from build123d import *

# Parameters (mm, degrees)
F0_R     = 2.157429
F0_R_2   = 5.60947
F1_DEPTH = 3.175
F2_DEPTH = 0.004921
F3_DEPTH = 3.175


with BuildPart() as f1:
    # F0 (on Front) → F1 (new body)
    with BuildSketch(Plane.XZ):
        with BuildLine():
            Line((19.481216, 38.301506), (-40.142396, 38.301506))
            ThreePointArc((-40.142396, 38.301506), (-44.686392, 36.387111), (-46.490546, 31.798229))
            Line((-46.490546, 31.798229), (-44.625234, 18.579618))
            ThreePointArc((-44.625234, 18.579618), (-43.776004, 17.017098), (-42.110151, 16.394528))
            Line((-42.110151, 16.394528), (21.620648, 16.394528))
            ThreePointArc((21.620648, 16.394528), (23.297675, 17.026865), (24.139706, 18.609033))
            Line((24.139706, 18.609033), (25.823629, 31.641185))
            ThreePointArc((25.823629, 31.641185), (24.07975, 36.330545), (19.481216, 38.301506))
        make_face()
        with Locations((-36.75957, 20.633117)):
            Circle(F0_R, mode=Mode.SUBTRACT)
        with Locations((17.996946, 20.940602)):
            Circle(F0_R, mode=Mode.SUBTRACT)
        with Locations((-38.274463, 31.951506)):
            Circle(F0_R_2, mode=Mode.SUBTRACT)
        with BuildLine():
            Line((-29.799683, 20.633117), (-29.799683, 34.853889))
            ThreePointArc((-29.799683, 34.853889), (-27.878732, 36.660702), (-26.0331, 34.777018))
            Line((-26.0331, 34.777018), (-26.0331, 20.556246))
            ThreePointArc((-26.0331, 20.556246), (-27.954051, 18.749433), (-29.799683, 20.633117))
        make_face(mode=Mode.SUBTRACT)
        with BuildLine():
            Line((-24.176236, 20.709988), (-24.176236, 34.93076))
            ThreePointArc((-24.176236, 34.93076), (-22.255285, 36.737572), (-20.409653, 34.853889))
            Line((-20.409653, 34.853889), (-20.409653, 20.633116))
            ThreePointArc((-20.409653, 20.633116), (-22.330604, 18.826304), (-24.176236, 20.709988))
        make_face(mode=Mode.SUBTRACT)
        with BuildLine():
            Line((-18.419787, 20.786859), (-18.419787, 35.007631))
            ThreePointArc((-18.419787, 35.007631), (-16.498836, 36.814444), (-14.653204, 34.93076))
            Line((-14.653204, 34.93076), (-14.653204, 20.709988))
            ThreePointArc((-14.653204, 20.709988), (-16.574155, 18.903175), (-18.419787, 20.786859))
        make_face(mode=Mode.SUBTRACT)
        with BuildLine():
            Line((-12.493486, 20.86373), (-12.493486, 35.084503))
            ThreePointArc((-12.493486, 35.084503), (-10.572535, 36.891315), (-8.726902, 35.007631))
            Line((-8.726902, 35.007631), (-8.726902, 20.786859))
            ThreePointArc((-8.726902, 20.786859), (-10.647853, 18.980047), (-12.493486, 20.86373))
        make_face(mode=Mode.SUBTRACT)
        with BuildLine():
            Line((-6.886294, 20.940602), (-6.886294, 35.161374))
            ThreePointArc((-6.886294, 35.161374), (-4.965343, 36.968187), (-3.11971, 35.084503))
            Line((-3.11971, 35.084503), (-3.11971, 20.86373))
            ThreePointArc((-3.11971, 20.86373), (-5.040661, 19.056918), (-6.886294, 20.940602))
        make_face(mode=Mode.SUBTRACT)
        with BuildLine():
            Line((-1.18931, 21.017473), (-1.18931, 35.238246))
            ThreePointArc((-1.18931, 35.238246), (0.73164, 37.045058), (2.577273, 35.161374))
            Line((2.577273, 35.161374), (2.577273, 20.940602))
            ThreePointArc((2.577273, 20.940602), (0.656322, 19.133789), (-1.18931, 21.017473))
        make_face(mode=Mode.SUBTRACT)
        with BuildLine():
            Line((4.431474, 21.017473), (4.431474, 35.238246))
            ThreePointArc((4.431474, 35.238246), (6.352424, 37.045058), (8.198057, 35.161374))
            Line((8.198057, 35.161374), (8.198057, 20.940602))
            ThreePointArc((8.198057, 20.940602), (6.277106, 19.133789), (4.431474, 21.017473))
        make_face(mode=Mode.SUBTRACT)
        with Locations((17.949626, 31.951506)):
            Circle(F0_R_2, mode=Mode.SUBTRACT)
    extrude(amount=F1_DEPTH)

    # F0 (on Front) → F2 (join)
    with BuildSketch(Plane.XZ):
        with BuildLine():
            Line((19.481216, 38.301506), (-40.142396, 38.301506))
            ThreePointArc((-40.142396, 38.301506), (-44.686392, 36.387111), (-46.490546, 31.798229))
            Line((-46.490546, 31.798229), (-44.625234, 18.579618))
            ThreePointArc((-44.625234, 18.579618), (-43.776004, 17.017098), (-42.110151, 16.394528))
            Line((-42.110151, 16.394528), (21.620648, 16.394528))
            ThreePointArc((21.620648, 16.394528), (23.297675, 17.026865), (24.139706, 18.609033))
            Line((24.139706, 18.609033), (25.823629, 31.641185))
            ThreePointArc((25.823629, 31.641185), (24.07975, 36.330545), (19.481216, 38.301506))
        make_face()
        with Locations((-36.75957, 20.633117)):
            Circle(F0_R, mode=Mode.SUBTRACT)
        with Locations((17.996946, 20.940602)):
            Circle(F0_R, mode=Mode.SUBTRACT)
        with Locations((-38.274463, 31.951506)):
            Circle(F0_R_2, mode=Mode.SUBTRACT)
        with BuildLine():
            Line((-29.799683, 20.633117), (-29.799683, 34.853889))
            ThreePointArc((-29.799683, 34.853889), (-27.878732, 36.660702), (-26.0331, 34.777018))
            Line((-26.0331, 34.777018), (-26.0331, 20.556246))
            ThreePointArc((-26.0331, 20.556246), (-27.954051, 18.749433), (-29.799683, 20.633117))
        make_face(mode=Mode.SUBTRACT)
        with BuildLine():
            Line((-24.176236, 20.709988), (-24.176236, 34.93076))
            ThreePointArc((-24.176236, 34.93076), (-22.255285, 36.737572), (-20.409653, 34.853889))
            Line((-20.409653, 34.853889), (-20.409653, 20.633116))
            ThreePointArc((-20.409653, 20.633116), (-22.330604, 18.826304), (-24.176236, 20.709988))
        make_face(mode=Mode.SUBTRACT)
        with BuildLine():
            Line((-18.419787, 20.786859), (-18.419787, 35.007631))
            ThreePointArc((-18.419787, 35.007631), (-16.498836, 36.814444), (-14.653204, 34.93076))
            Line((-14.653204, 34.93076), (-14.653204, 20.709988))
            ThreePointArc((-14.653204, 20.709988), (-16.574155, 18.903175), (-18.419787, 20.786859))
        make_face(mode=Mode.SUBTRACT)
        with BuildLine():
            Line((-12.493486, 20.86373), (-12.493486, 35.084503))
            ThreePointArc((-12.493486, 35.084503), (-10.572535, 36.891315), (-8.726902, 35.007631))
            Line((-8.726902, 35.007631), (-8.726902, 20.786859))
            ThreePointArc((-8.726902, 20.786859), (-10.647853, 18.980047), (-12.493486, 20.86373))
        make_face(mode=Mode.SUBTRACT)
        with BuildLine():
            Line((-6.886294, 20.940602), (-6.886294, 35.161374))
            ThreePointArc((-6.886294, 35.161374), (-4.965343, 36.968187), (-3.11971, 35.084503))
            Line((-3.11971, 35.084503), (-3.11971, 20.86373))
            ThreePointArc((-3.11971, 20.86373), (-5.040661, 19.056918), (-6.886294, 20.940602))
        make_face(mode=Mode.SUBTRACT)
        with BuildLine():
            Line((-1.18931, 21.017473), (-1.18931, 35.238246))
            ThreePointArc((-1.18931, 35.238246), (0.73164, 37.045058), (2.577273, 35.161374))
            Line((2.577273, 35.161374), (2.577273, 20.940602))
            ThreePointArc((2.577273, 20.940602), (0.656322, 19.133789), (-1.18931, 21.017473))
        make_face(mode=Mode.SUBTRACT)
        with BuildLine():
            Line((4.431474, 21.017473), (4.431474, 35.238246))
            ThreePointArc((4.431474, 35.238246), (6.352424, 37.045058), (8.198057, 35.161374))
            Line((8.198057, 35.161374), (8.198057, 20.940602))
            ThreePointArc((8.198057, 20.940602), (6.277106, 19.133789), (4.431474, 21.017473))
        make_face(mode=Mode.SUBTRACT)
        with Locations((17.949626, 31.951506)):
            Circle(F0_R_2, mode=Mode.SUBTRACT)
    extrude(amount=F2_DEPTH)

    # F0 (on Front) → F3 (join)
    with BuildSketch(Plane.XZ):
        with BuildLine():
            Line((19.481216, 38.301506), (-40.142396, 38.301506))
            ThreePointArc((-40.142396, 38.301506), (-44.686392, 36.387111), (-46.490546, 31.798229))
            Line((-46.490546, 31.798229), (-44.625234, 18.579618))
            ThreePointArc((-44.625234, 18.579618), (-43.776004, 17.017098), (-42.110151, 16.394528))
            Line((-42.110151, 16.394528), (21.620648, 16.394528))
            ThreePointArc((21.620648, 16.394528), (23.297675, 17.026865), (24.139706, 18.609033))
            Line((24.139706, 18.609033), (25.823629, 31.641185))
            ThreePointArc((25.823629, 31.641185), (24.07975, 36.330545), (19.481216, 38.301506))
        make_face()
        with Locations((-36.75957, 20.633117)):
            Circle(F0_R, mode=Mode.SUBTRACT)
        with Locations((17.996946, 20.940602)):
            Circle(F0_R, mode=Mode.SUBTRACT)
        with Locations((-38.274463, 31.951506)):
            Circle(F0_R_2, mode=Mode.SUBTRACT)
        with BuildLine():
            Line((-29.799683, 20.633117), (-29.799683, 34.853889))
            ThreePointArc((-29.799683, 34.853889), (-27.878732, 36.660702), (-26.0331, 34.777018))
            Line((-26.0331, 34.777018), (-26.0331, 20.556246))
            ThreePointArc((-26.0331, 20.556246), (-27.954051, 18.749433), (-29.799683, 20.633117))
        make_face(mode=Mode.SUBTRACT)
        with BuildLine():
            Line((-24.176236, 20.709988), (-24.176236, 34.93076))
            ThreePointArc((-24.176236, 34.93076), (-22.255285, 36.737572), (-20.409653, 34.853889))
            Line((-20.409653, 34.853889), (-20.409653, 20.633116))
            ThreePointArc((-20.409653, 20.633116), (-22.330604, 18.826304), (-24.176236, 20.709988))
        make_face(mode=Mode.SUBTRACT)
        with BuildLine():
            Line((-18.419787, 20.786859), (-18.419787, 35.007631))
            ThreePointArc((-18.419787, 35.007631), (-16.498836, 36.814444), (-14.653204, 34.93076))
            Line((-14.653204, 34.93076), (-14.653204, 20.709988))
            ThreePointArc((-14.653204, 20.709988), (-16.574155, 18.903175), (-18.419787, 20.786859))
        make_face(mode=Mode.SUBTRACT)
        with BuildLine():
            Line((-12.493486, 20.86373), (-12.493486, 35.084503))
            ThreePointArc((-12.493486, 35.084503), (-10.572535, 36.891315), (-8.726902, 35.007631))
            Line((-8.726902, 35.007631), (-8.726902, 20.786859))
            ThreePointArc((-8.726902, 20.786859), (-10.647853, 18.980047), (-12.493486, 20.86373))
        make_face(mode=Mode.SUBTRACT)
        with BuildLine():
            Line((-6.886294, 20.940602), (-6.886294, 35.161374))
            ThreePointArc((-6.886294, 35.161374), (-4.965343, 36.968187), (-3.11971, 35.084503))
            Line((-3.11971, 35.084503), (-3.11971, 20.86373))
            ThreePointArc((-3.11971, 20.86373), (-5.040661, 19.056918), (-6.886294, 20.940602))
        make_face(mode=Mode.SUBTRACT)
        with BuildLine():
            Line((-1.18931, 21.017473), (-1.18931, 35.238246))
            ThreePointArc((-1.18931, 35.238246), (0.73164, 37.045058), (2.577273, 35.161374))
            Line((2.577273, 35.161374), (2.577273, 20.940602))
            ThreePointArc((2.577273, 20.940602), (0.656322, 19.133789), (-1.18931, 21.017473))
        make_face(mode=Mode.SUBTRACT)
        with BuildLine():
            Line((4.431474, 21.017473), (4.431474, 35.238246))
            ThreePointArc((4.431474, 35.238246), (6.352424, 37.045058), (8.198057, 35.161374))
            Line((8.198057, 35.161374), (8.198057, 20.940602))
            ThreePointArc((8.198057, 20.940602), (6.277106, 19.133789), (4.431474, 21.017473))
        make_face(mode=Mode.SUBTRACT)
        with Locations((17.949626, 31.951506)):
            Circle(F0_R_2, mode=Mode.SUBTRACT)
    extrude(amount=F3_DEPTH)


solid = f1.part
Input: part model. Units: mm. Frame: model coordinates. A direction names the side the tool comes from. Give positions to 0.01 mm unless a question says otherwise; leave off trailing zeros. Loops run counter-clockwise (first coordinate to the right, second up) from the corner with the lowest first, then second, coordinate; pieces in that order, holes last. Notation, with made-up numbers: (1, -34) -> (55, -34) arc R27 ccw to (55, -14) -> close; hole circle Ø6 at (78, 28.25). An arc over 180 degrees is marked (long way). Answer as a JSON object with one key per item and string values. Group by question number.
Item 1: Line query: probe 1 along Z at (x, y) = (18, -1.05); probe 2 along Z at (x, y) = (-35.5, -1.95); probe 3 along Z at (x, y) = (-29, -2.55). Output: solid intervals per line, ascending.
Item 2: Cut plane B-B, the plane x = -29. Return the cut outline in (y, z) (1 decimal).
Item 3: Reachability of faces 1 (the flat face through (-12.493, -2, 28)), 2 (the flat face through (-11, -2, 16.395)) from +Z, -Z, +X, -X, +Y, -Y: full face, straight path, thin tool, end or side. Return the list, or none.
Item 4: Cut plane A-A, the plane z = 25. State how many separate pieces and enclosed holes the cut face has, and give its area (3 significant figures).
Item 5: Pin query (flat end, axial travel): P1, Ø1, axis at y = -1.5, z = 29, coming from the +X side; P2, Ø1.6, axis at y = -1.5, z = 29.5, coming from the +X side; P3, Ø1.5, axis at y = -0.5, z = 24, coming from the -X side. Return the tip coordinate at first contact, or that it passes through.
Item 6: Pull-direction query (X, two-part tool) for faces 3 (the flat face through (-18.42, -2, 28)), 4 (the cylindrical face through (-44.637, -1.565, 36.438)), 5 (the cylindrical face through (-22.296, -1.565, 36.738)), 6 (the flat face through (-2.8, 0, 27.5)); classes: released by +X, released by -X, zero draft, split by the parting line, or undercut.
Checks:
{
 "1": {"probe 1": "z = 16.39 to 18.78, 23.1 to 26.34, 37.56 to 38.3", "probe 2": "z = 16.39 to 18.88, 22.38 to 27.08, 36.83 to 38.3", "probe 3": "z = 16.39 to 19.09, 36.32 to 38.3"},
 "2": {"outline": "(-3.2, 16.4) -> (0, 16.4) -> (0, 19.1) -> (-3.2, 19.1) -> close; (-3.2, 36.3) -> (0, 36.3) -> (0, 38.3) -> (-3.2, 38.3) -> close"},
 "3": {"face 1": "+Y, -Y", "face 2": "-Z, +X, -X, +Y, -Y"},
 "4": {"separate pieces": "8", "enclosed holes": "0", "area": "140 mm²"},
 "5": {"P1": "stops at x = 25.55", "P2": "stops at x = 25.65", "P3": "stops at x = -45.5"},
 "6": {"face 3": "undercut", "face 4": "released by -X", "face 5": "undercut", "face 6": "zero draft"}
}
